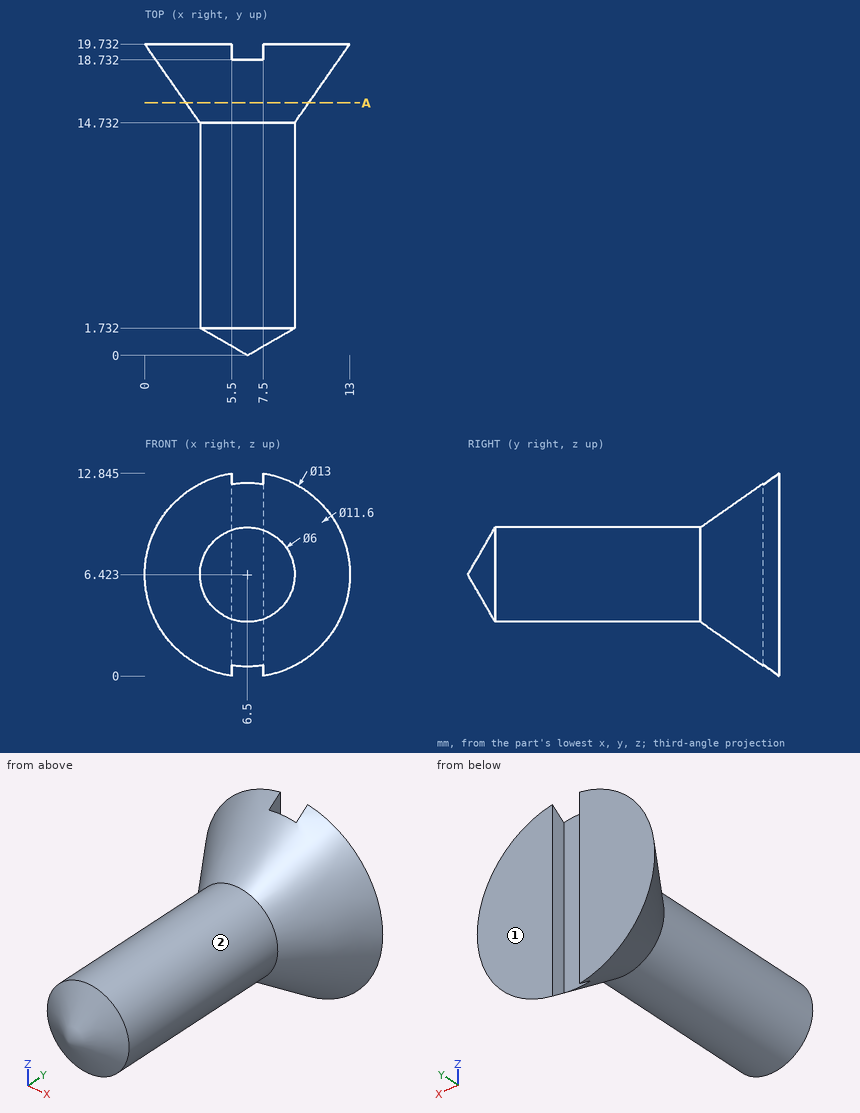
Input: dimensioned drawing with shaded views. Units: mm. Origin: part minimum x, y, z. A direction names the side the tool comes from. Give positions to 0.01 mm unless a question says otherwise; leave off trailing zeros. Write each loop counter-clockwise with the first axis right and the second up, starting at its lowest first coordinate (ties: lowest second). Pieces come first, ordered by that corner, then holes. Notation, with made-up numbers: (45, 83) - (66, 83) arc R31 ccw to (66, 114) - close; hole circle Ø9 at (-2, -40). An arc over 180 degrees is marked (long way). One line per item, written item: value. Start each with the question number.
Q1. Set-up query: the marked faces 1 and 2. Return all of +Z, -Z, +X, -X, +Y, -Y with unobstructed straight access to the full face (end or side cutting, diameter ignored); none if empty.
Q2. Section query A-A, the plane y = 16. Return the cut outline in (x, z) (1 decimal).
Q3. First-contact query: pin 1 Ø2 at (x, y) = (8.5, 2) entering from +Z; pin 2 Ø0.5 at (y, z) = (19, 6) entering from -X; pin 3 Ø4 at (x, z) = (5, 1.5) entering from -Y. Flat tips, straight axial feed; report the tip coordinate or a pass-through.
Q4. Material intervals for probe 1 along X at (y, z) = (9.25, 7) (1 decimal); probe 2 along Y at (x, z) = (9.75, 3.75) (1 decimal); probe 3 along Z at (x, y) = (4.5, 4) (1 decimal), sorted ascending. Write a range as from..to.
Answer:
1. face 1: +Z, -Z, +X, -X, +Y
1. face 2: -Y
2. outline: circle Ø7.8 at (6.5, 6.4)
3. pin 1: stops at z = 9.25
3. pin 2: stops at x = 0.35
3. pin 3: stops at y = 14.94
4. probe 1: x = 3.6..9.4
4. probe 2: y = 16.5..19.7
4. probe 3: z = 4.2..8.7
